```python
from build123d import *

# Parameters (mm, degrees)
BOSS_EXTRUDE1_DEPTH     = 3.175
SKETCH3_R               = 1.27
CUT_EXTRUDE1_DEPTH      = 96.302901976
CUT_EXTRUDE2_DEPTH      = 96.302901976
CUT_EXTRUDE2_DEPTH_BACK = 96.302901976
FILLET1_R               = 12.7


with BuildPart() as part:
    # Sketch2 → Boss-Extrude1 (new body)
    with BuildSketch(Plane(origin=(0, 0, 0), x_dir=(1, 0, 0), z_dir=(0, 1, 0))):
        with BuildLine():
            Line((6.35, 63.5), (57.15, 63.5))
            Line((57.15, 63.5), (57.15, -63.5))
            Line((57.15, -63.5), (12.7, -63.5))
            ThreePointArc((12.7, -63.5), (0, -76.2), (-12.7, -63.5))
            Line((-12.7, -63.5), (-57.15, -63.5))
            Line((-57.15, -63.5), (-57.15, 63.5))
            Line((-57.15, 63.5), (-6.35, 63.5))
            Line((-6.35, 63.5), (-6.35, -57.15))
            Line((-6.35, -57.15), (6.35, -57.15))
            Line((6.35, -57.15), (6.35, 63.5))
        make_face()
    extrude(amount=BOSS_EXTRUDE1_DEPTH)

    # Sketch3 → Cut-Extrude1 (cut, through all)
    with BuildSketch(Plane(origin=(0, 3.175, 0), x_dir=(1, 0, 0), z_dir=(0, 1, 0))):
        with Locations(Location((0, -69.85, 0), (0, 0, 270))):
            Circle(SKETCH3_R)
    extrude(amount=-CUT_EXTRUDE1_DEPTH, mode=Mode.SUBTRACT)

    # Sketch4 → Cut-Extrude2 (cut, two sides: drawn at the far end of the back side and taken through both)
    with BuildSketch(Plane(origin=(0, 3.175, 0), x_dir=(1, 0, 0), z_dir=(0, 1, 0)).offset(-CUT_EXTRUDE2_DEPTH_BACK)):
        with BuildLine():
            Line((-57.15, -63.5), (-12.7, -63.5))
            Line((-12.7, -63.5), (-12.7, -55.798007597))
            ThreePointArc((-12.7, -55.798007597), (-40.162037001, -41.837402835), (-57.15, -16.137771034))
            Line((-57.15, -16.137771034), (-57.15, -63.5))
        make_face()
        with BuildLine():
            Line((-57.15, 63.5), (-57.15, 22.487771034))
            ThreePointArc((-57.15, 22.487771034), (-37.70568739, 50.264136363), (-6.35, 63.164858518))
            Line((-6.35, 63.164858518), (-6.35, 63.5))
            Line((-6.35, 63.5), (-57.15, 63.5))
        make_face()
        with BuildLine():
            Line((57.15, -63.5), (57.15, -16.137771034))
            ThreePointArc((57.15, -16.137771034), (40.162037001, -41.837402835), (12.7, -55.798007597))
            Line((12.7, -55.798007597), (12.7, -63.5))
            Line((12.7, -63.5), (57.15, -63.5))
        make_face()
        with BuildLine():
            Line((57.15, 63.5), (6.35, 63.5))
            Line((6.35, 63.5), (6.35, 63.164858518))
            ThreePointArc((6.35, 63.164858518), (37.70568739, 50.264136363), (57.15, 22.487771034))
            Line((57.15, 22.487771034), (57.15, 63.5))
        make_face()
    extrude(amount=CUT_EXTRUDE2_DEPTH + CUT_EXTRUDE2_DEPTH_BACK, mode=Mode.SUBTRACT)

    # Fillet1
    fillet1_edges = [part.edges().sort_by_distance(p)[0] for p in [
        (12.7, 1.5875, 55.798007597),
        (-12.7, 1.5875, 55.798007597),
    ]]
    fillet(fillet1_edges, radius=FILLET1_R)


solid = part.part
```
Can you work these out from the model? Positions are in its coordinate system, mm. A direction names the side the tool comes from. Coordinates: 2 decimals unless noted, no trailing zeros. Order: outer loops, then holes, each group sorted by start corner. A loop starts at its lowest first (then second) coordinate and runs counter-clockwise, first axis right, second up. Notation, with made-up numbers: (1, 61.25) - (46, 61.25) arc R23 ccw to (46, 97.25) - close; hole circle Ø4 at (-25, 0). An arc over 180 degrees is marked (long way). Answer in a Markdown table with one row per item.
1. Suppose I cut it at D-D (x = -43.5). Please give me the cut outline in (y, z) (3 decimals).
Reply:
| item | result |
|---|---|
| outline | (0, -44.97) - (3.175, -44.97) - (3.175, 38.62) - (0, 38.62) - close |
2. Suppose I cut it at B-B (z = 29.5). Please give me the cut outline in (x, y) (3 decimals).
Reply:
| item | result |
|---|---|
| outline | (-50.709, 0) - (-6.35, 0) - (-6.35, 3.175) - (-50.709, 3.175) - close; (6.35, 0) - (50.709, 0) - (50.709, 3.175) - (6.35, 3.175) - close |
3. Suppose I cut it at A-A (z = 5.5). Please give me the cut outline in (x, y) (3 decimals), and give its area (3 significant figures).
Reply:
| item | result |
|---|---|
| outline | (-57.15, 0) - (-6.35, 0) - (-6.35, 3.175) - (-57.15, 3.175) - close; (6.35, 0) - (57.15, 0) - (57.15, 3.175) - (6.35, 3.175) - close |
| area | 323 mm^2 |
4. For faces 4 (the flat face through (-12, 0, 6)), 5 (the flat face through (0, 2, 57.15)), which set-ups out of +Z, -Z, +X, -X, +Y, -Y let a thin tool reach every point of the face, with its end or its side?
Reply:
| item | result |
|---|---|
| face 4 | +Z, -Z, +X, -X, -Y |
| face 5 | -Z, +Y, -Y |
5. If I drill on line 1 along X through (y, z) = (0.9, -20.5); line 2 along X through (y, z) = (0.85, 69.85); line 3 along Z through (x, y) = (28.5, 2.95), over which ranges is the centre line in solid material (lowest first)?
Reply:
| item | result |
|---|---|
| line 1 | x = -57.15 to -6.35, 6.35 to 57.15 |
| line 2 | x = -11 to -1.27, 1.27 to 11 |
| line 3 | z = -56.34 to 49.99 |
6. Suppose I cut it at C-C (x = 49). Please give me the cut outline in (y, z) (3 decimals), and give its area (3 significant figures).
Reply:
| item | result |
|---|---|
| outline | (0, -38.362) - (3.175, -38.362) - (3.175, 32.012) - (0, 32.012) - close |
| area | 223 mm^2 |
7. If we mould it in two halves opening along X, with no side actions, what happens to faces 1 (the flat face through (6.35, 2, -2)), 2 (the cylindrical face through (0.267, 1.565, 76.197)), 3 (the flat face through (-12, 3.175, 6))? For each: pulls with the +X half, pulls with the -X half, needs draft (parallel to the pull), parting line crosses it, or undercut.
Reply:
| item | result |
|---|---|
| face 1 | undercut |
| face 2 | parting line crosses it |
| face 3 | needs draft |
8. For pin 1 (1 mm diameter, centred on x = -2, y = 2, fed in from -Z); pin 2 (1 mm diameter, centred on y = 1, z = 30, fed in from +X), each with a flat end and sliding along its axis, tell me the tip position at first contact or that it passes through.
Reply:
| item | result |
|---|---|
| pin 1 | stops at z = 57.15 |
| pin 2 | stops at x = 50.71 |
